Source: CAD feature listing. Evaluate the final solid. Frame: model axes, mm. Coordinates: 2 decimals unless noted, no trailing zeros. Order: outer loops, then holes, each group sorted by start corner. A loop starts at its lowest first (then second) coordinate and runs counter-clockwise, first axis right, second up. Notation, with made-up numbers: (-33.75, -10) -> (-22.75, -10) arc R11 ccw to (-22.75, 1) -> close; hole circle Ø6 at (72.5, -34.75). An arc over 180 degrees is marked (long way). Write item = value, one per line. Start each with the question number.
Item 1: Contact query for flat-ended pins moving along their axis: pin 1 (10 mm diameter, centred on x = -29, y = -6, fed in from +Z); pin 2 (4 mm diameter, centred on x = -45, z = 22, fed in from +Y); pin 3 (5 mm diameter, centred on x = 5.5, y = -16.5, fed in from +Z); pin 4 (10 mm diameter, centred on x = 10.5, y = -19, fed in from -Z). Output: stop coordinate, or through.
Item 2: Section query B-B (z = 39.5). Output: boundary loops of the cut face in (x, y).
Item 3: Section query D-D (y = -16.75). Output: boundary loops of the cut face in (x, z) (3 decimals), then the cut area to 3 significant figures.
Item 4: Section query A-A (x = 26). Output: boundary loops of the cut face in (y, z).
Item 5: Section query C-C (z = 59). Output: boundary loops of the cut face in (x, y).
Item 6: Mould query, pull axis Z, two halves, no side actions, for faces 1 (the cylindrical face through (-0.85, -12.522, 68.394)), 2 (the flat face through (-59.7, -12.5, -1.9)), 3 (the cylindrical face through (-1.03, -12.52, 50.79)), 4 (the flat face through (-63.5, -13, 29)). Classes: released by +Z, released by -Z, zero draft, split by the parting line, or undercut.
Item 7: Ray query, line 1 along X through (y, z) = (-8.5, 29.5); line 2 along X through (y, z) = (-23.25, 19.5); line 3 along Z through (x, y) = (11, -4). Return the intervals inside material, ascending. Write a range as [from, to].
```python
from build123d import *

# Parameters (mm, degrees)
F1_DEPTH = 25.4


with BuildPart() as f1:
    # F0 (on Front) → F1 (new body)
    with BuildSketch(Plane.XZ):
        with BuildLine():
            Line((-63.5, 0), (-57.15, 0))
            Line((-57.15, 0), (-57.15, 50.8))
            ThreePointArc((-57.15, 50.8), (0, 68.3973958737), (57.15, 50.8))
            Line((57.15, 50.8), (57.15, 57.15))
            ThreePointArc((57.15, 57.15), (-3.175, 76.495759208), (-63.5, 57.15))
            Line((-63.5, 57.15), (-63.5, 0))
        make_face()
        with BuildLine():
            ThreePointArc((-50.8, -6.35), (-46.3098719395, -4.4901280605), (-44.45, 0))
            Line((-44.45, 0), (-50.8, 0))
            ThreePointArc((-50.8, 0), (-50.700684167, 3.175), (-50.403125, 6.3375855209))
            ThreePointArc((-50.403125, 6.3375855209), (-55.1475478002, 4.6283180665), (-57.15, 0))
            ThreePointArc((-57.15, 0), (-56.8241389426, -2.0080463142), (-55.88, -3.81))
            Line((-55.88, -3.81), (-50.8, -6.35))
        make_face()
        with BuildLine():
            ThreePointArc((-57.15, 0), (-55.1475478002, 4.6283180665), (-50.403125, 6.3375855209))
            ThreePointArc((-50.403125, 6.3375855209), (0, 50.8), (50.403125, 6.3375855209))
            ThreePointArc((50.403125, 6.3375855209), (55.1475478002, 4.6283180665), (57.15, 0))
            ThreePointArc((57.15, 0), (0, 57.15), (-57.15, 0))
        make_face()
        with BuildLine():
            Line((-50.8, 0), (-44.45, 0))
            ThreePointArc((-44.45, 0), (-46.1716819335, 4.3475478002), (-50.403125, 6.3375855209))
            ThreePointArc((-50.403125, 6.3375855209), (-50.700684167, 3.175), (-50.8, 0))
        make_face()
        with BuildLine():
            ThreePointArc((50.403125, 6.3375855209), (46.1716819335, 4.3475478002), (44.45, 0))
            Line((44.45, 0), (50.8, 0))
            ThreePointArc((50.8, 0), (50.700684167, 3.175), (50.403125, 6.3375855209))
        make_face()
        with BuildLine():
            Line((50.8, 0), (44.45, 0))
            ThreePointArc((44.45, 0), (50.8, -6.35), (57.15, 0))
            ThreePointArc((57.15, 0), (55.1475478002, 4.6283180665), (50.403125, 6.3375855209))
            ThreePointArc((50.403125, 6.3375855209), (50.700684167, 3.175), (50.8, 0))
        make_face()
        with BuildLine():
            Line((-63.5, 0), (-55.88, -3.81))
            ThreePointArc((-55.88, -3.81), (-56.8241389426, -2.0080463142), (-57.15, 0))
            Line((-57.15, 0), (-63.5, 0))
        make_face()
        with BuildLine():
            ThreePointArc((-55.88, -3.81), (-53.6398063314, -5.6796126628), (-50.8, -6.35))
            Line((-50.8, -6.35), (-55.88, -3.81))
        make_face()
    extrude(amount=F1_DEPTH)


solid = f1.part
```
Computed:
q1.pin_1 = 74.38
q1.pin_2 = 0
q1.pin_3 = 76.31
q1.pin_4 = 48.38
q2.outline = (-63.5, -25.4) -> (-57.15, -25.4) -> (-57.15, 0) -> (-63.5, 0) -> close; (-41.3, -25.4) -> (-31.94, -25.4) -> (-31.94, 0) -> (-41.3, 0) -> close; (31.94, -25.4) -> (41.3, -25.4) -> (41.3, 0) -> (31.94, 0) -> close
q3.outline = (-63.5, 0) -> (-55.88, -3.81) arc R6.35 ccw (long way) to (-50.403, 6.338) arc R50.8 cw to (50.403, 6.338) arc R6.35 ccw (long way) to (57.15, 0) arc R57.15 ccw to (-57.15, 0) -> (-57.15, 50.8) arc R101.6 cw to (57.15, 50.8) -> (57.15, 57.15) arc R103.727 ccw to (-63.5, 57.15) -> close
q3.area = 2,590 mm^2
q4.outline = (-25.4, 43.64) -> (0, 43.64) -> (0, 50.89) -> (-25.4, 50.89) -> close; (-25.4, 65.01) -> (0, 65.01) -> (0, 72.31) -> (-25.4, 72.31) -> close
q5.outline = (-60.82, -25.4) -> (-42.68, -25.4) -> (-42.68, 0) -> (-60.82, 0) -> close; (42.68, -25.4) -> (54.47, -25.4) -> (54.47, 0) -> (42.68, 0) -> close
q6.face_1 = undercut
q6.face_2 = released by -Z
q6.face_3 = undercut
q6.face_4 = zero draft
q7.line_1 = [-63.5, -57.15], [-48.95, -41.36], [41.36, 48.95]
q7.line_2 = [-63.5, -57.15], [-53.72, -46.91], [46.91, 53.72]
q7.line_3 = [49.59, 56.08], [67.8, 75.52]
